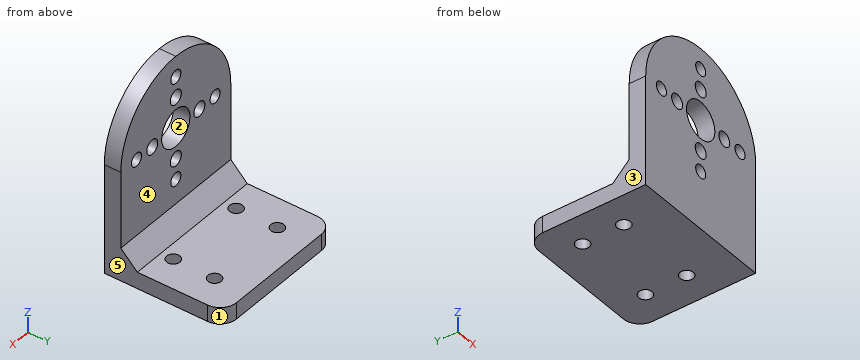
from build123d import *

# Parameters (mm, degrees)
SKETCH_1_W          = 35
SKETCH_1_H          = 44
EXTRUDE_1_DEPTH     = 4
SKETCH_2_W          = 35
SKETCH_2_H          = 4
EXTRUDE_2_DEPTH     = 25
SKETCH_3_R          = 4.5
SKETCH_3_R_2        = 1.75
SKETCH_3_R_3        = 1.6
CUT_EXTRUDE_1_DEPTH = 20
CHAMFER_1_SIZE      = 4
SKETCH_5_R          = 1.6
CUT_EXTRUDE_2_DEPTH = 20
FILLET_1_R          = 17.5
FILLET_2_R          = 4


with BuildPart() as part:
    # 草图1 → 凸台-拉伸1 (new body)
    with BuildSketch(Plane(origin=(0, 0, 0), x_dir=(1, 0, 0), z_dir=(0, 1, 0))):
        with Locations((17.5, 22)):
            Rectangle(SKETCH_1_W, SKETCH_1_H)
    extrude(amount=EXTRUDE_1_DEPTH)

    # 草图2 → 凸台-拉伸2 (add)
    with BuildSketch(Plane(origin=(0, 4, 0), x_dir=(1, 0, 0), z_dir=(0, 1, 0))):
        with Locations((17.5, 42)):
            Rectangle(SKETCH_2_W, SKETCH_2_H)
    extrude(amount=EXTRUDE_2_DEPTH)

    # 草图3 → 切除-拉伸1 (cut)
    with BuildSketch(Plane(origin=(0, 4, 0), x_dir=(1, 0, 0), z_dir=(0, 1, 0))):
        with Locations(Location((17.5, 17.5, 0), (0, 0, 270))):
            Circle(SKETCH_3_R)
        with Locations(Location((17.5, 25, 0), (0, 0, 270))):
            Circle(SKETCH_3_R_2)
        with Locations(Location((25, 17.5, 0), (0, 0, 270))):
            Circle(SKETCH_3_R_2)
        with Locations(Location((10, 17.5, 0), (0, 0, 270))):
            Circle(SKETCH_3_R_2)
        with Locations(Location((17.5, 10, 0), (0, 0, 270))):
            Circle(SKETCH_3_R_2)
        with Locations(Location((17.5, 30, 0), (0, 0, 270))):
            Circle(SKETCH_3_R_3)
        with Locations(Location((30, 17.5, 0), (0, 0, 270))):
            Circle(SKETCH_3_R_3)
        with Locations(Location((17.5, 5, 0), (0, 0, 270))):
            Circle(SKETCH_3_R_3)
        with Locations(Location((5, 17.5, 0), (0, 0, 270))):
            Circle(SKETCH_3_R_3)
    extrude(amount=-CUT_EXTRUDE_1_DEPTH, mode=Mode.SUBTRACT)

    # 倒角1
    chamfer_1_edges = [part.edges().sort_by_distance(p)[0] for p in [
        (17.5, 4, -40),
    ]]
    chamfer(chamfer_1_edges, length=CHAMFER_1_SIZE)

    # 草图5 → 切除-拉伸2 (cut)
    with BuildSketch(Plane.XY.offset(-40)):
        with Locations((7.5, 21)):
            Circle(SKETCH_5_R)
        with Locations((27.5, 21)):
            Circle(SKETCH_5_R)
        with Locations((27.5, 11)):
            Circle(SKETCH_5_R)
        with Locations((7.5, 11)):
            Circle(SKETCH_5_R)
    extrude(amount=-CUT_EXTRUDE_2_DEPTH, mode=Mode.SUBTRACT)

    # 圆角1
    fillet_1_edges = [part.edges().sort_by_distance(p)[0] for p in [
        (35, 2, 0),
        (0, 2, 0),
    ]]
    fillet(fillet_1_edges, radius=FILLET_1_R - 0.0001)  # a hair under: the kernel refuses the full size

    # 圆角2
    fillet_2_edges = [part.edges().sort_by_distance(p)[0] for p in [
        (0, 29, -42),
        (35, 29, -42),
    ]]
    fillet(fillet_2_edges, radius=FILLET_2_R)


solid = part.part
Could you check a few things on this model? Use its own coordinates, in mm. Face numbers are marked on the shaded views. A direction names the side the tool comes from. Give positions to 0.01 mm unless a question says otherwise; leave off trailing zeros. Loops run counter-clockwise (first coordinate to the right, second up) from the corner with the lowest first, then second, coordinate; pieces in that order, holes last. Notation, with made-up numbers: M -5.75,2.25 L 28.25,2.25 A19 ccw 28.25,27.25 Z; hole C 79.5,-39 d1. An arc over 180 degrees is marked long. Answer as a JSON object with one key per item and string values.
Q1. Suppose I cut it at A-A, the plane z = -30. List the corners of the cut face in (x, y) for me.
Values found:
{"outline": "M 0,0 L 15.9,0 L 15.9,4 L 0,4 Z; M 19.1,0 L 35,0 L 35,4 L 19.1,4 Z"}
Q2. For the marked faces 4 and 5, which set-ups out of +Z, -Z, +X, -X, +Y, -Y let a thin tool reach every point of the face, with its end or its side?
Values found:
{"face 4": "+Z, +X, -X, +Y", "face 5": "+Z, -Z, +X, +Y, -Y"}
Q3. If we mould it in two halves opening along X, with no side actions, what happens to the marked faces 1, 2 and 3? For each: pulls with the +X half, pulls with the -X half, needs draft (parallel to the pull), parting line crosses it, or undercut.
Values found:
{"face 1": "pulls with the +X half", "face 2": "undercut", "face 3": "pulls with the -X half"}
Q4. Suppose I cut it at C-C, the plane x = 27.5. List the corners of the cut face in (y, z) for me.
Values found:
{"outline": "M 0,-44 L 9.4,-44 L 9.4,-40 L 8,-40 L 4,-36 L 4,-3.14 L 0,-3.14 Z; M 12.6,-44 L 19.4,-44 L 19.4,-40 L 12.6,-40 Z; M 22.6,-44 L 29,-44 L 29,-40 L 22.6,-40 Z"}
Q5. Suppose I cut it at D-D, the plane x = 20. List the corners of the cut face in (y, z) for me.
Values found:
{"outline": "M 0,-44 L 29,-44 L 29,-40 L 8,-40 L 4,-36 L 4,-21.24 L 0,-21.24 Z; M 0,-13.76 L 4,-13.76 L 4,-0.18 L 0,-0.18 Z"}
Q6. Suppose I cut it at B-B, the plane y = 2. State how many separate pieces and enclosed holes the cut face has, plus the area to 3 significant figures.
Values found:
{"separate pieces": "1", "enclosed holes": "9", "area": "1,270 mm²"}
Q7. For P1, Ø5, axis at x = 16, y = 16.5, coming from the +Z side; P2, Ø8, axis at x = 17.5, z = -17.5, coming from the +Y side; P3, Ø12, axis at x = 10.5, z = -20.5, coming from the +Y side; P4, Ø17, axis at x = 20.5, y = 13.5, coming from the +Z side, each with a flat end and sliding along its axis, tell me the tip position at first contact or that it passes through.
Values found:
{"P1": "stops at z = -40", "P2": "passes through", "P3": "stops at y = 4", "P4": "stops at z = -37"}
Q8. If I drill on probe 1 along X at (y, z) = (3, -17.5); probe 2 along Y at (x, z) = (27.5, -43.2); probe 3 along Z at (x, y) = (16.5, 1), over which ranges is the centre line in solid material (lowest first)? Write a range as [from, to].
Values found:
{"probe 1": "x = [0, 3.4], [6.6, 8.25], [11.75, 13], [22, 23.25], [26.75, 28.4], [31.6, 35]", "probe 2": "y = [0, 9.4], [12.6, 19.4], [22.6, 29]", "probe 3": "z = [-44, -31.25], [-28.75, -26.44], [-23.56, -21.89], [-13.11, -11.44], [-8.56, -6.25], [-3.75, -0.03]"}
